Design review of the part built by this model. Coordinates are the model's own, in mm. Round coordinates to 2 decimals unless told otherwise and drop trailing zeros. Loops run counter-clockwise (first coordinate to the right, second up) from the corner with the lowest first, then second, coordinate; pieces in that order, holes last. Notation, with made-up numbers: (22, 8.5) -> (60, 8.5) arc R25 ccw to (60, 25.5) -> close; hole circle Ø10 at (-10, 56). An arc over 180 degrees is marked (long way). Write each question's results on one line, items separated by ' | '. Start each with the question number.
from build123d import *

# Parameters (mm, degrees)
SALIENTE_EXTRUIR2_DEPTH = 1.5
CROQUIS5_R              = 34.003076767
CROQUIS5_R_2            = 3.25
SALIENTE_EXTRUIR3_DEPTH = 1.5
CORTAR_EXTRUIR6_DEPTH   = 1.5
REDONDEO2_R             = 0.65
CORTAR_EXTRUIR7_START   = -1.5
CORTAR_EXTRUIR7_DEPTH   = 1.5
REDONDEO3_R             = 0.65
CORTAR_EXTRUIR8_START   = -1.5
CORTAR_EXTRUIR8_DEPTH   = 1.5
REDONDEO4_R             = 0.65
CROQUIS9_R              = 2.5
CORTAR_EXTRUIR10_DEPTH  = 49.111001436


with BuildPart() as part:
    # Croquis3 → Saliente-Extruir2 (new body)
    with BuildSketch(Plane.XY):
        with BuildLine():
            Line((-5.157307796, -27.019308404), (-6.280793024, -32.905285166))
            ThreePointArc((-6.280793024, -32.905285166), (-6.494024336, -33.227196877), (-6.872990522, -33.301219661))
            ThreePointArc((-6.872990522, -33.301219661), (0, 34.003076767), (6.872990522, -33.301219661))
            ThreePointArc((6.872990522, -33.301219661), (6.494024336, -33.227196877), (6.280793024, -32.905285166))
            Line((6.280793024, -32.905285166), (5.157307796, -27.019308404))
            ThreePointArc((5.157307796, -27.019308404), (0, -22.753293006), (-5.157307796, -27.019308404))
        make_face()
    extrude(amount=SALIENTE_EXTRUIR2_DEPTH)

    # Croquis5 → Saliente-Extruir3 (add)
    with BuildSketch(Plane.XY):
        with Locations(Location((0, 0, 0), (0, 0, 180))):
            Circle(CROQUIS5_R)
        with Locations((0, -28.003709015)):
            Circle(CROQUIS5_R_2, mode=Mode.SUBTRACT)
    extrude(amount=SALIENTE_EXTRUIR3_DEPTH)

    # Croquis4 → Cortar-Extruir6 (cut)
    with BuildSketch(Plane.XY):
        with BuildLine():
            ThreePointArc((10.940986169, 30.28750526), (17.262989212, 27.1850576), (22.759447155, 22.782574886))
            Line((22.759447155, 22.782574886), (24.031592832, 24.056013293))
            ThreePointArc((24.031592832, 24.056013293), (18.227908832, 28.704574012), (11.552535657, 31.980433854))
            Line((11.552535657, 31.980433854), (10.940986169, 30.28750526))
        make_face()
    extrude(amount=CORTAR_EXTRUIR6_DEPTH, mode=Mode.SUBTRACT)

    # Redondeo2
    redondeo2_edges = [part.edges().sort_by_distance(p)[0] for p in [
        (11.552535657, 31.980433854, 0.75),
        (10.940986169, 30.28750526, 0.75),
        (22.759447155, 22.782574886, 0.75),
        (24.031592832, 24.056013293, 0.75),
    ]]
    fillet(redondeo2_edges, radius=REDONDEO2_R)

    # Croquis6 → Cortar-Extruir7 (cut)
    with BuildSketch(Plane.XY.offset(1.5).offset(CORTAR_EXTRUIR7_START)):
        with BuildLine():
            Line((-24.137163622, 21.312844303), (-25.488752409, 22.506282018))
            ThreePointArc((-25.488752409, 22.506282018), (-19.986507056, 27.509066965), (-13.528288511, 31.196067694))
            Line((-13.528288511, 31.196067694), (-12.8109257, 29.541837835))
            ThreePointArc((-12.8109257, 29.541837835), (-18.926685124, 26.050347219), (-24.137163622, 21.312844303))
        make_face()
    extrude(amount=CORTAR_EXTRUIR7_DEPTH, mode=Mode.SUBTRACT)

    # Redondeo3
    redondeo3_edges = [part.edges().sort_by_distance(p)[0] for p in [
        (-12.8109257, 29.541837835, 0.75),
        (-24.137163622, 21.312844303, 0.75),
        (-25.488752409, 22.506282018, 0.75),
        (-13.528288511, 31.196067694, 0.75),
    ]]
    fillet(redondeo3_edges, radius=REDONDEO3_R)

    # Croquis7 → Cortar-Extruir8 (cut)
    with BuildSketch(Plane.XY.offset(1.5).offset(CORTAR_EXTRUIR8_START)):
        with BuildLine():
            Line((-13.67660573, -30.301073746), (-13.98863049, -30.992377234))
            ThreePointArc((-13.98863049, -30.992377234), (-13.286060557, -31.299997196), (-12.57673119, -31.59169293))
            Line((-12.57673119, -31.59169293), (-12.296199688, -30.887021347))
            ThreePointArc((-12.296199688, -30.887021347), (-12.699963864, -29.919239916), (-13.67660573, -30.301073746))
        make_face()
    extrude(amount=CORTAR_EXTRUIR8_DEPTH, mode=Mode.SUBTRACT)

    # Redondeo4
    redondeo4_edges = [part.edges().sort_by_distance(p)[0] for p in [
        (-12.57673119, -31.59169293, 0.75),
        (-13.98863049, -30.992377234, 0.75),
    ]]
    fillet(redondeo4_edges, radius=REDONDEO4_R)

    # Croquis9 → Cortar-Extruir10 (cut, through all)
    with BuildSketch(Plane.XY):
        with Locations((-22.9496732, -13.25)):
            Circle(CROQUIS9_R)
        with Locations((22.9496732, -13.25)):
            Circle(CROQUIS9_R)
        with Locations((0, 26.5)):
            Circle(CROQUIS9_R)
    extrude(amount=CORTAR_EXTRUIR10_DEPTH, mode=Mode.SUBTRACT)


solid = part.part
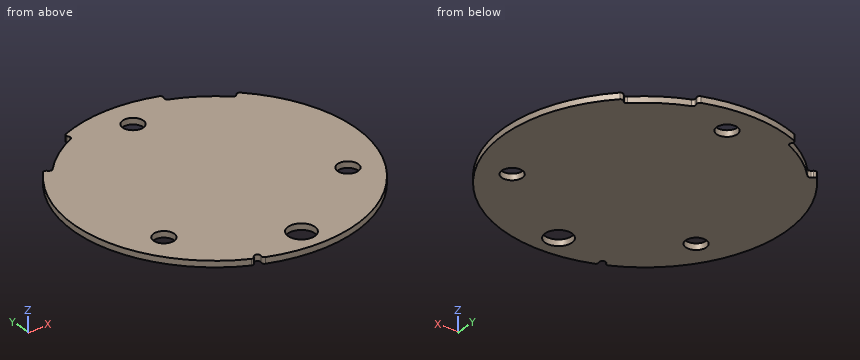
1) Take a section at D-D (x = -22.5). Write out the cut boundary in (y, z), plus the area to 3 significant figures.
2) Take a section at A-A (x = 0). Write out the cut boundary in (y, z).
3) To check wall thickness, follow line 1 (Y direction, x = 0, z = 0.75); line 2 (X direction, y = -13.25, z = 1.05); line 3 (X direction, y = 1, z = 0.9). State the ranges of each line that lie inside material, in increasing order. Write a range as from..to.
4) Insertion check: pin 1 (8 mm diameter, centred on x = -22.95, y = -13.25, fed in from -Z). The pin has a flat end and moves straight along its axis. Give the tip position at first contact, or say it passes through.
5) Take a section at B-B (y = -13.25). Write out the cut boundary in (x, z), plus the area to 3 significant figures.
6) Take a section at C-C (z = 0.8). Write out the cut boundary in (x, y), plus the area to 3 significant figures.
Geometry check:
1) outline: (-25.49, 0) -> (-15.71, 0) -> (-15.71, 1.5) -> (-25.49, 1.5) -> close; (-10.79, 0) -> (23.03, 0) -> (23.03, 1.5) -> (-10.79, 1.5) -> close | area: 65.4 mm^2
2) outline: (-34, 0) -> (-31.25, 0) -> (-31.25, 1.5) -> (-34, 1.5) -> close; (-24.75, 0) -> (24, 0) -> (24, 1.5) -> (-24.75, 1.5) -> close; (29, 0) -> (34, 0) -> (34, 1.5) -> (29, 1.5) -> close
3) line 1: y = -34..-31.25, -24.75..24, 29..34 | line 2: x = -31.32..-25.45, -20.45..20.45, 25.45..31.32 | line 3: x = -33.99..33.99
4) pin 1: stops at z = 0
5) outline: (-31.32, 0) -> (-25.45, 0) -> (-25.45, 1.5) -> (-31.32, 1.5) -> close; (-20.45, 0) -> (20.45, 0) -> (20.45, 1.5) -> (-20.45, 1.5) -> close; (25.45, 0) -> (31.32, 0) -> (31.32, 1.5) -> (25.45, 1.5) -> close | area: 78.9 mm^2
6) outline: (-25.92, 22.01) arc R34 ccw to (-14.59, -30.71) arc R0.65 ccw to (-13.72, -30.39) -> (-13.68, -30.3) arc R0.75 cw to (-12.3, -30.89) -> (-12.33, -30.98) arc R0.65 ccw to (-11.96, -31.83) arc R34 ccw to (24.5, 23.58) arc R0.65 ccw to (23.57, 23.59) -> (23.21, 23.24) arc R0.65 cw to (22.3, 23.23) arc R32.2 ccw to (11.54, 30.07) arc R0.65 cw to (11.16, 30.89) -> (11.33, 31.36) arc R0.65 ccw to (10.93, 32.2) arc R34 ccw to (-12.92, 31.45) arc R0.65 ccw to (-13.27, 30.59) -> (-13.07, 30.13) arc R0.65 cw to (-13.39, 29.28) arc R32.2 ccw to (-23.71, 21.79) arc R0.65 cw to (-24.62, 21.74) -> (-25, 22.07) arc R0.65 ccw to start; hole circle Ø5 at (-22.95, -13.25); hole circle Ø6.5 at (0, -28); hole circle Ø5 at (0, 26.5); hole circle Ø5 at (22.95, -13.25) | area: 3,490 mm^2
